Design review of the part built by this model. Coordinates are the model's own, in mm. A direction names the side the tool comes from. Coordinates: 2 decimals unless noted, no trailing zeros. Loops run counter-clockwise (first coordinate to the right, second up) from the corner with the lowest first, then second, coordinate; pieces in that order, holes last. Notation, with made-up numbers: M -12.75,8 L 29.25,8 A25 ccw 29.25,35 Z; hole C -24,-7.5 d7. An arc over 180 degrees is marked long. Put each result on its own line as item: value. Start each with the question number.
(1) Take a section at A-A, the plane z = 7.5. Give the boundary of the cut face in (x, y).
(2) Clearance check with flat-ended pins moving along their axes: pin 1 (4 mm diameter, centred on x = -35, y = 1, fed in from +Z); pin 2 (1.5 mm diameter, centred on y = -1, z = 12, fed in from +X); pin 3 (3 mm diameter, centred on x = -24, z = 21.5, fed in from +Y). State where each tip first meets the part, or that it passes through.
(3) For faces 1 (the cylindrical face through (-14.5, 1.05, 15.72)), 2 (the flat face through (-29, 0, 0)), list the 3-axis set-ups (+Z, -Z, +X, -X, +Y, -Y) from which the entire face can be reached by the end or side of a thin tool; tool diameter is ignored.
(4) For probe 1 along Z at (x, y) = (-31, 2.25); probe 2 along Y at (x, z) = (-40.5, 5.25); probe 3 along X at (y, z) = (-2.75, 4), list the stretches that pass through material, from the lowest coordinate up. Write a range as [from, to].
```python
from build123d import *

# Parameters (mm, degrees)
F0_R     = 3.5
F1_DEPTH = 6
F1_TAPER = -3
F2_DEPTH = 25
F3_R     = 0.7


with BuildPart() as f1:
    # F0 (on Top) → F1 (new body)
    with BuildSketch(Plane.XY):
        with BuildLine():
            Line((-17.214833647, 4.9607837082), (-36.902333647, 7.4411755624))
            ThreePointArc((-36.902333647, 7.4411755624), (-45.339833647, 0), (-36.902333647, -7.4411755624))
            Line((-36.902333647, -7.4411755624), (-17.214833647, -4.9607837082))
            ThreePointArc((-17.214833647, -4.9607837082), (-12.839833647, 0), (-17.214833647, 4.9607837082))
        make_face()
        Polygon((-36.080574115, 3.3148663974), (-34.0894453707, 0.1338697521), (-35.8487049027, -3.1809966452), (-39.599093179, -3.3148663974), (-41.5902219233, -0.1338697521), (-39.8309623913, 3.1809966452), align=None, mode=Mode.SUBTRACT)
        with Locations((-17.839833647, 0)):
            Circle(F0_R, mode=Mode.SUBTRACT)
    extrude(amount=F1_DEPTH, taper=F1_TAPER)

    # F0 (on Top) → F2 (join)
    with BuildSketch(Plane.XY):
        with Locations((-17.839833647, 0)):
            Circle(F0_R)
    extrude(amount=F2_DEPTH)

    # F3
    f3_edges = [f1.edges().sort_by_distance(p)[0] for p in [
        (-27.058584, 6.20098, 0),
        (-45.339834, 0, 0),
        (-27.058584, -6.20098, 0),
        (-12.839834, 0, 0),
        (-40.594658, -1.724368, 0),
        (-40.710592, 1.523563, 0),
        (-37.955768, 3.247932, 0),
        (-35.08501, 1.724368, 0),
        (-34.969075, -1.523563, 0),
        (-37.723899, -3.247932, 0),
        (-27.019278, 6.51296, 6),
        (-45.65428, 0, 6),
        (-27.019278, -6.51296, 6),
        (-12.525387, 0, 6),
        (-21.339834, 0, 6),
        (-40.328121, -1.557531, 6),
        (-37.735116, -2.933685, 6),
        (-40.432838, 1.376154, 6),
        (-35.246829, -1.376154, 6),
        (-37.944551, 2.933685, 6),
        (-35.351547, 1.557531, 6),
    ]]
    fillet(f3_edges, radius=F3_R)


solid = f1.part
```
Computed values:
1. outline: C -17.84,0 d7
2. pin 1: stops at z = 6
2. pin 2: stops at x = -14.35
2. pin 3: passes through
3. face 1: +Z
3. face 2: -Z, +X, -X, +Y, -Y
4. probe 1: z = [0, 6]
4. probe 2: y = [-7.31, -1.36], [1.33, 7.31]
4. probe 3: x = [-45.04, -39.71], [-35.86, -13.42]
